from build123d import *

# Parameters (mm, degrees)
BOSS_EXTRUDE1_DEPTH = 21
SKETCH2_R           = 9
CUT_EXTRUDE1_DEPTH  = 20


with BuildPart() as part:
    # Sketch1 → Boss-Extrude1 (new, symmetric)
    with BuildSketch(Plane.XY):
        Polygon((0, 0), (-60, 0), (-60, 30), (-15, 50), (0, 50), align=None)
    extrude(amount=BOSS_EXTRUDE1_DEPTH, both=True)

    # Sketch2 → Cut-Extrude1 (cut, symmetric)
    with BuildSketch(Plane(origin=(0, 0, 0), x_dir=(0, 0, -1), z_dir=(1, 0, 0))):
        with Locations(Location((0, 25, 0), (0, 0, 90))):
            Circle(SKETCH2_R)
    extrude(amount=CUT_EXTRUDE1_DEPTH, both=True, mode=Mode.SUBTRACT)


solid = part.part
Read the model definition and answer for the solid it produces. Units are mm, in the model's axes. Round coordinates to 2 decimals unless told otherwise and drop trailing zeros. Write each loop counter-clockwise with the first axis right and the second up, starting at its lowest first coordinate (ties: lowest second). Pieces come first, ordered by that corner, then holes.
Q1. Find section D-D on z = 0. Determine the outline of the cut face in (x, y).
Values:
outline: (-60, 0) - (0, 0) - (0, 16) - (-20, 16) - (-20, 34) - (0, 34) - (0, 50) - (-15, 50) - (-60, 30) - close
Q2. Find section A-A on x = -4. Determine the outline of the cut face in (y, z).
Values:
outline: (0, -21) - (50, -21) - (50, 21) - (0, 21) - close; hole circle Ø18 at (25, 0)
Q3. Find section C-C on y = 25. Determine the outline of the cut face in (x, z).
Values:
outline: (-60, -21) - (0, -21) - (0, -9) - (-20, -9) - (-20, 9) - (0, 9) - (0, 21) - (-60, 21) - close
Q4. Find section B-B on z = -12. Determine the outline of the cut face in (x, y).
Values:
outline: (-60, 0) - (0, 0) - (0, 50) - (-15, 50) - (-60, 30) - close
Q5. Straight lines are drawn through the part: line 1 (Z direction, x = -12.25, y = 25); line 2 (X direction, y = 20, z = -6); line 3 (Y direction, x = -16.5, z = -3). For each, find the intervals that lie inside material, in ascending order.
Values:
line 1: z = -21 to -9, 9 to 21
line 2: x = -60 to -20
line 3: y = 0 to 16.51, 33.49 to 49.33
Q6. The mould has two halves that part along Y. Classify faces 1 (the face through (-20, 25, 0)), 2 (the face through (-8, 50, 0)), 3 (the face through (-9.86, 33.584, 2.703)), 4 (the face through (-30, 20, -21)): released by +Y, released by -Y, zero draft, split by the parting line, or undercut.
Values:
face 1: undercut
face 2: released by +Y
face 3: undercut
face 4: zero draft
